```python
from build123d import *

# Parameters (mm, degrees)
F0_W      = 73.615912
F0_H      = 44.880818
F1_DEPTH  = 50.8
F2_R      = 10.722735
F2_R_2    = 14.315515
F3_DEPTH  = 25.4
F4_R      = 5.08
F5_DEPTH  = 25.4
F6_R      = 10.061194
F7_DEPTH  = 25.4
F8_R      = 7.163215
F9_DEPTH  = 25.4
F10_W     = 19.266809
F10_H     = 16.048783
F11_DEPTH = 25.4


with BuildPart() as f1:
    # F0 (on Top) → F1 (new body)
    with BuildSketch(Plane.XY):
        with Locations((3.049085, -1.806261)):
            Rectangle(F0_W, F0_H)
    extrude(amount=F1_DEPTH)

    # F2 (on face) → F3 (cut)
    with BuildSketch(Plane.XY.offset(50.8)):
        with Locations((-15.909195, 0)):
            Circle(F2_R)
        with Locations((21.110246, 0)):
            Circle(F2_R_2)
    extrude(amount=-F3_DEPTH, mode=Mode.SUBTRACT)

    # F4 (on face) → F5 (join)
    with BuildSketch(Plane.XY.offset(50.8)):
        with Locations((0, -10.984484)):
            Circle(F4_R)
    extrude(amount=F5_DEPTH)

    # F6 (on face) → F7 (cut)
    with BuildSketch(Plane.XZ.offset(24.24667)):
        with Locations((0, 28.342469)):
            Circle(F6_R)
    extrude(amount=-F7_DEPTH, mode=Mode.SUBTRACT)

    # F8 (on face) → F9 (cut)
    with BuildSketch(Plane.XZ.offset(24.24667)):
        with Locations((30.216709, 28.516769)):
            Circle(F8_R)
    extrude(amount=-F9_DEPTH, mode=Mode.SUBTRACT)

    # F10 (on face) → F11 (join)
    with BuildSketch(Plane.XZ.offset(24.24667)):
        with Locations((-24.125466, 8.024392)):
            Rectangle(F10_W, F10_H)
    extrude(amount=F11_DEPTH)


solid = f1.part
```
Could you check a few things on this model? Use its own coordinates, in mm. A direction names the side the tool comes from. Coordinates: 2 decimals unless noted, no trailing zeros. Loops run counter-clockwise (first coordinate to the right, second up) from the corner with the lowest first, then second, coordinate; pieces in that order, holes last.
1) Will these pins go through, and if not, where does the flat tip stop? pin 1 Ø6 at (x, z) = (-1, 30.5) entering from -Y; pin 2 Ø17 at (x, y) = (-13, 5) entering from +Z; pin 3 Ø4 at (x, y) = (-22, -34.5) entering from +Z.
Reported:
pin 1: stops at y = 1.15
pin 2: stops at z = 50.8
pin 3: stops at z = 16.05
2) Imagine slicing it at B-B (x = -28). List the corners of the cut face in (y, z) for me.
Reported:
outline: (-49.65, 0) - (20.63, 0) - (20.63, 50.8) - (-24.25, 50.8) - (-24.25, 16.05) - (-49.65, 16.05) - close
3) Which directions (+Z, -Z, +X, -X, +Y, -Y) give clear straight access to the entire face, cutting with the end or side of a thin tool? Please do faces 1 (the face through (3, 20.634, 25)), 2 (the face through (-23.81, 7.25, 38.28)), 3 (the face through (32, 1.153, 25)).
Reported:
face 1: +Z, -Z, +X, -X, +Y
face 2: +Z
face 3: -Y
4) Imagine slicing it at D-D (x = 0). List the corners of the cut face in (y, z) for me, and give its area (3 significant figures).
Reported:
outline: (-24.25, 0) - (20.63, 0) - (20.63, 50.8) - (-5.9, 50.8) - (-5.9, 76.2) - (-16.06, 76.2) - (-16.06, 50.8) - (-24.25, 50.8) - (-24.25, 38.4) - (1.15, 38.4) - (1.15, 18.28) - (-24.25, 18.28) - close
area: 2,030 mm2
5) Imagine slicing it at A-A (y = 0). List the corners of the cut face in (x, z) for me, and give its area (3 significant figures).
Reported:
outline: (-33.76, 0) - (39.86, 0) - (39.86, 50.8) - (35.43, 50.8) - (35.43, 33.43) arc R7.16 cw (long way) to (23.77, 25.4) - (9.62, 25.4) arc R10.06 cw to (-9.62, 25.4) - (-26.63, 25.4) - (-26.63, 50.8) - (-33.76, 50.8) - close; (-5.19, 36.96) arc R10.06 cw to (6.79, 35.76) - (6.79, 50.8) - (-5.19, 50.8) - close
area: 2,170 mm2
6) Please list where these lines run through material, in increasing order: line 1 along X through (y, z) = (0, 45.25); line 2 along X through (y, z) = (0, 34); line 3 along X through (y, z) = (-20.5, 31).
Reported:
line 1: x = -33.76 to -26.63, -5.19 to 6.79, 35.43 to 39.86
line 2: x = -33.76 to -26.63, 35.43 to 39.86
line 3: x = -33.76 to -9.7, 9.7 to 23.5, 36.94 to 39.86
7) Thinking about a two-plate mould opening in X: for faces 4 (the face through (4.643, -11.724, 19.416)), 5 (the face through (-24, -37, 16.049)), 6 (the face through (-33.759, -2, 25)), which applies, released by +X, released by -X, zero draft, split by the parting line, or undercut?
Reported:
face 4: undercut
face 5: zero draft
face 6: released by -X
8) Imagine slicing it at C-C (z = 12). List the corners of the cut face in (x, y) for me, and give its area (3 significant figures).
Reported:
outline: (-33.76, -49.65) - (-14.49, -49.65) - (-14.49, -24.25) - (39.86, -24.25) - (39.86, 20.63) - (-33.76, 20.63) - close
area: 3,790 mm2
